```python
from build123d import *

# Parameters (mm, degrees)
F0_W     = 30
F0_H     = 30
F1_DEPTH = 457.2
F2_R     = 8.052642
F2_R_2   = 8.052679
F3_DEPTH = 30.001
F5_W     = 30
F5_H     = 27.321835
F6_DEPTH = 203.2


with BuildPart() as f1:
    # F0 (on Front) → F1 (new body)
    with BuildSketch(Plane.XZ):
        with Locations((15, 15)):
            Rectangle(F0_W, F0_H)
    extrude(amount=F1_DEPTH)

    # F2 (on face) → F3 (cut, through all)
    with BuildSketch(Plane.XY.offset(30)):
        with Locations((16.058933, -303.081602)):
            Circle(F2_R)
        with Locations((14.143813, -69.052368)):
            Circle(F2_R_2)
    extrude(amount=-F3_DEPTH, mode=Mode.SUBTRACT)

    # F5 (on face) → F6 (join)
    with BuildSketch(Plane.XY.offset(30)):
        with Locations((15, -214.939082)):
            Rectangle(F5_W, F5_H)
    extrude(amount=F6_DEPTH)

    # F7: F1 across plane


with BuildPart() as f1_1:
    add(f1.part)
    add(f1.part.mirror(Plane(origin=(14.996897, -229.902144, 233.2), x_dir=(1, 0, 0), z_dir=(0, 0, 1))))


solid = f1_1.part
```
Here's how the part is built. I have some questions about the finished solid (model axes, mm). A direction names the side the tool comes from. Give positions to 0.01 mm unless a question says otherwise; leave off trailing zeros. Order: outer loops, then holes, each group sorted by start corner. A loop starts at its lowest first (then second) coordinate and runs counter-clockwise, first axis right, second up. Notation, with made-up numbers: M 78.5,-15 L 111.5,-15 A32 cw 111.5,24 Z; hole C 62.5,40 d4. An arc over 180 degrees is marked long. Use a Markdown table: item, result. Add a question column.
1. For pin 1 Ø9 at (x, z) = (11.5, 194) entering from +Y; pin 2 Ø1.5 at (x, z) = (3.5, 177.5) entering from -Y, each with a flat end and sliding along its axis, tell me the tip position at first contact or that it passes through.
2. Suppose I cut it at A-A (y = -238.5). List the corners of the cut face in (x, z) for me.
3. Suppose I cut it at C-C (z = 194.5). List the corners of the cut face in (x, y) for me.
4. I need wall thicknesses on probe 1 along Z at (x, y) = (26.5, -357.5); probe 2 along Y at (x, z) = (10.25, 421). Which ranges of each line are inside material? Lowest first, please. Write a range as from..to.
5. On a 3-axis mill with a long thin cutter (end or side, diameter ignored), from which of +Z, -Z, +X, -X, +Y, -Y can I reach the whole of each face in a straight line? I mean faces 1 (the flat face through (0, -211, 234)), 2 (the flat face through (15, -228.6, 236)), 3 (the flat face through (15, -99, 30)). Say none if no direction works.
6. If we mould it in two halves opening along Y, with no side actions, what happens to faces 4 (the cylindrical face through (17.86, -76.196, 15.21)), 5 (the flat face through (15, -457.2, 451)), 6 (the flat face through (15, -99, 436.4))? For each: +Y half, -Y half, draft (parallel to the pull), parting line (faces both ways), or undercut.
7. Suppose I cut it at B-B (x = 13.5). List the corners of the cut face in (y, z) for me, and give its area (3 significant figures).
Results list:
| question | item | result |
|---|---|---|
| 1 | pin 1 | stops at y = -201.28 |
| 1 | pin 2 | stops at y = -228.6 |
| 2 | outline | M 0,0 L 30,0 L 30,30 L 0,30 Z; M 0,436.4 L 30,436.4 L 30,466.4 L 0,466.4 Z |
| 3 | outline | M 0,-228.6 L 30,-228.6 L 30,-201.28 L 0,-201.28 Z |
| 4 | probe 1 | z = 0..30, 436.4..466.4 |
| 4 | probe 2 | y = -228.6..-201.28 |
| 5 | face 1 | +Z, -Z, -X, +Y, -Y |
| 5 | face 2 | +X, -X, -Y |
| 5 | face 3 | +X, -X, +Y |
| 6 | face 4 | undercut |
| 6 | face 5 | -Y half |
| 6 | face 6 | draft |
| 7 | outline | M -457.2,0 L -310.72,0 L -310.72,30 L -457.2,30 Z; M -457.2,436.4 L -310.72,436.4 L -310.72,466.4 L -457.2,466.4 Z; M -295.45,0 L -77.08,0 L -77.08,30 L -201.28,30 L -201.28,436.4 L -77.08,436.4 L -77.08,466.4 L -295.45,466.4 L -295.45,436.4 L -228.6,436.4 L -228.6,30 L -295.45,30 Z; M -61.03,0 L 0,0 L 0,30 L -61.03,30 Z; M -61.03,436.4 L 0,436.4 L 0,466.4 L -61.03,466.4 Z |
| 7 | area | 36,700 mm² |
